```python
from build123d import *

# Parameters (mm, degrees)
SKETCH1_W                        = 25.4
SKETCH1_H                        = 25.4
SKETCH1_W_2                      = 19.05
SKETCH1_H_2                      = 19.05
BOSS_EXTRUDE1_DEPTH              = 241.3
F_10_0_1935_DIAMETER_HOLE1_D     = 4.9149
F_10_0_1935_DIAMETER_HOLE1_DEPTH = 50.8
F_10_0_1935_DIAMETER_HOLE1_TIP   = 1.476584928
SKETCH5_R                        = 2.464210786
CUT_EXTRUDE1_DEPTH               = 243.965306165
SKETCH6_W                        = 25.4
SKETCH6_H                        = 63.5
CUT_EXTRUDE2_DEPTH               = 243.965306165


with BuildPart() as part:
    # Sketch1 → Boss-Extrude1 (new, symmetric)
    with BuildSketch(Plane.XY):
        Rectangle(SKETCH1_W, SKETCH1_H)
        Rectangle(SKETCH1_W_2, SKETCH1_H_2, mode=Mode.SUBTRACT)
    extrude(amount=BOSS_EXTRUDE1_DEPTH, both=True)

    # #10 (0.1935) Diameter Hole1
    with Locations(Plane(origin=(0, 12.7, 0), x_dir=(1, 0, 0), z_dir=(0, 1, 0))):
        with Locations((0, -228.6), (0, 88.9), (0, 114.3), (0, 139.7), (0, 165.1), (0, 190.5), (0, 215.9)):
            Hole(F_10_0_1935_DIAMETER_HOLE1_D / 2, depth=F_10_0_1935_DIAMETER_HOLE1_DEPTH)
            with Locations((0, 0, -(F_10_0_1935_DIAMETER_HOLE1_DEPTH + F_10_0_1935_DIAMETER_HOLE1_TIP / 2))):  # 118° drill point
                Cone(0, F_10_0_1935_DIAMETER_HOLE1_D / 2, F_10_0_1935_DIAMETER_HOLE1_TIP, mode=Mode.SUBTRACT)

    # Sketch5 → Cut-Extrude1 (cut, through all)
    with BuildSketch(Plane(origin=(0, 12.7, 0), x_dir=(1, 0, 0), z_dir=(0, 1, 0))):
        with Locations(Location((-0.70643934, -165.103929701, 0), (0, 0, 180))):
            Circle(SKETCH5_R)
    extrude(amount=-CUT_EXTRUDE1_DEPTH, mode=Mode.SUBTRACT)

    # Sketch6 → Cut-Extrude2 (cut, through all)
    with BuildSketch(Plane(origin=(0, 12.7, 0), x_dir=(1, 0, 0), z_dir=(0, 1, 0))):
        with Locations((0, 209.55)):
            Rectangle(SKETCH6_W, SKETCH6_H)
    extrude(amount=-CUT_EXTRUDE2_DEPTH, mode=Mode.SUBTRACT)


solid = part.part
```
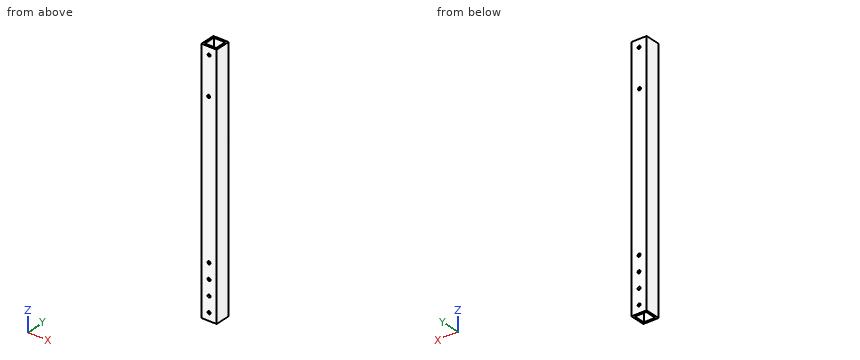
For this review, take the finished solid that the model builds, in its own axes (mm). Coordinates: 2 decimals unless noted, no trailing zeros. Loops run counter-clockwise (first coordinate to the right, second up) from the corner with the lowest first, then second, coordinate; pieces in that order, holes last. Notation, with made-up numbers: (62, -18) - (114, -18) arc R30 cw to (114, 21) - close; hole circle Ø2 at (-34.75, 27.5). An arc over 180 degrees is marked (long way). Use one line per item in the form item = value. Start each with the question number.
1) To check wall thickness, follow probe 1 along X at (y, z) = (-11.55, 228.6); probe 2 along X at (y, z) = (6.75, 11) (3 decimals). State the ranges of each line that lie inside material, in increasing order. Write a range as from..to.
2) For pin 1 (4 mm diameter, centred on x = 0, z = -139.7, fed in from +Y), flat-tipped, find the tip position at first contact; note if it passes through.
3) Take a section at A-A (y = 6). State the section outline as (x, z) points (3 decimals), plus the area to 3 significant figures.
4) Take a section at B-B (z = 57). State the section outline as (x, y) points (3 decimals).
From the geometry:
q1.probe_1 = -12.7..-2.46, 2.46..12.7
q1.probe_2 = -12.7..-9.525, 9.525..12.7
q2.pin_1 = through
q3.outline = (-12.7, -177.8) - (-9.525, -177.8) - (-9.525, 241.3) - (-12.7, 241.3) - close; (9.525, -177.8) - (12.7, -177.8) - (12.7, 241.3) - (9.525, 241.3) - close
q3.area = 2,660 mm2
q4.outline = (-12.7, -12.7) - (12.7, -12.7) - (12.7, 12.7) - (-12.7, 12.7) - close; hole (-9.525, -9.525) - (9.525, -9.525) - (9.525, 9.525) - (-9.525, 9.525) - close
